Can you work these out from the model? Positions are in its coordinate system, mm. Give positions to 0.01 mm unless a question says otherwise; leave off trailing zeros. Order: outer loops, then holes, each group sorted by start corner. A loop starts at its lowest first (then second) coordinate and runs counter-clockwise, first axis right, second up. Notation, with made-up numbers: M 13.25,-12 L 24.25,-12 A23 cw 24.25,-4 Z; hole C -28,-16 d5. An arc over 180 degrees is marked long. Use one line per item in the form item = value. Start each with the question number.
1. Will these pins go through, and if not, where does the flat tip stop? P1, Ø3, axis at x = 86.5, y = 63.5, coming from the -Z side; P2, Ø2.5, axis at x = 24, y = 24, coming from the -Z side.
2. I want a section at B-B, the plane z = 2.2. Count the separate pieces of the cut face and the enclosed holes in it, and give its area (3 significant figures).
3. I want a section at A-A, the plane x = 36. List the corners of the cut face in (y, z) for me, and give its area (3 significant figures).
4. I want a section at C-C, the plane y = 80.5. List the corners of the cut face in (x, z) for me.
5. I need wall thicknesses on L1, parallel to X at y = 63.55, z = 1.6; L2, parallel to Y at x = 72, z = 2.8; L3, parallel to Y at x = 85.55, z = 1.9. Which ranges of each line are inside material? Lowest first, please.
6. I want a section at D-D, the plane x = 68. List the corners of the cut face in (y, z) for me.
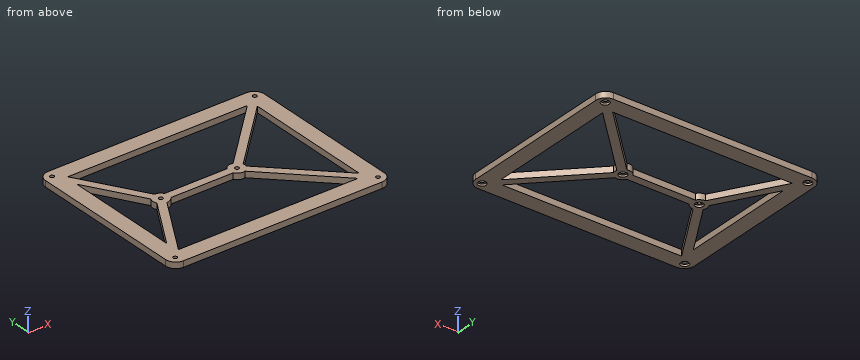
```python
from build123d import *

# Parameters (mm, degrees)
SKETCH002_R     = 1
PAD001_DEPTH    = 3
SKETCH003_R     = 2
POCKET001_DEPTH = 1


with BuildPart() as part:
    # Sketch002 → Pad001 (new body)
    with BuildSketch(Plane.XY):
        with BuildLine():
            Line((129.15, 25), (129.15, 102.15))
            ThreePointArc((129.15, 102.15), (127.685534, 105.685534), (124.15, 107.15))
            Line((124.15, 107.15), (25, 107.15))
            ThreePointArc((25, 107.15), (21.464466, 105.685534), (20, 102.15))
            Line((20, 102.15), (20, 25))
            ThreePointArc((20, 25), (21.464466, 21.464466), (25, 20))
            Line((25, 20), (124.15, 20))
            ThreePointArc((124.15, 20), (127.685534, 21.464466), (129.15, 25))
        make_face()
        with Locations((24, 103.15)):
            Circle(SKETCH002_R, mode=Mode.SUBTRACT)
        with Locations((24, 24)):
            Circle(SKETCH002_R, mode=Mode.SUBTRACT)
        with Locations((125.15, 24)):
            Circle(SKETCH002_R, mode=Mode.SUBTRACT)
        with Locations((125.15, 103.15)):
            Circle(SKETCH002_R, mode=Mode.SUBTRACT)
        with Locations((85.55, 63.55)):
            Circle(SKETCH002_R, mode=Mode.SUBTRACT)
        with Locations((47.5, 63.55)):
            Circle(SKETCH002_R, mode=Mode.SUBTRACT)
        with BuildLine():
            ThreePointArc((50.964102, 65.55), (49.479216, 67.026018), (47.452085, 67.549713))
            Line((28.699389, 99.15), (47.452085, 67.549713))
            Line((118.321573, 99.15), (28.699389, 99.15))
            Line((86.585276, 67.413703), (118.321573, 99.15))
            ThreePointArc((86.585276, 67.413703), (84.019266, 67.245518), (82.085898, 65.55))
            Line((50.964102, 65.55), (82.085898, 65.55))
        make_face(mode=Mode.SUBTRACT)
        with BuildLine():
            ThreePointArc((82.085898, 61.55), (84.020434, 59.853999), (86.587717, 59.686951))
            Line((118.314728, 28), (86.587717, 59.686951))
            Line((28.703156, 28), (118.314728, 28))
            Line((47.449866, 59.550314), (28.703156, 28))
            ThreePointArc((47.449866, 59.550314), (49.478252, 60.073433), (50.964102, 61.55))
            Line((50.964102, 61.55), (82.085898, 61.55))
        make_face(mode=Mode.SUBTRACT)
        with BuildLine():
            Line((89.414357, 62.517165), (121.15, 30.821592))
            Line((121.15, 30.821592), (121.15, 96.321573))
            Line((121.15, 96.321573), (89.413703, 64.585276))
            ThreePointArc((89.414357, 62.517165), (89.55, 63.551263), (89.413703, 64.585276))
        make_face(mode=Mode.SUBTRACT)
        with BuildLine():
            Line((44.012189, 65.508361), (28, 92.490603))
            Line((28, 92.490603), (28, 34.647227))
            Line((28, 34.647227), (44.011104, 61.593574))
            ThreePointArc((44.012189, 65.508361), (43.5, 63.551109), (44.011104, 61.593574))
        make_face(mode=Mode.SUBTRACT)
    extrude(amount=PAD001_DEPTH)

    # Sketch003 → Pocket001 (cut)
    with BuildSketch(Plane.XY):
        with Locations((24, 103.15)):
            Circle(SKETCH003_R)
        with Locations((24, 24)):
            Circle(SKETCH003_R)
        with Locations((125.15, 24)):
            Circle(SKETCH003_R)
        with Locations((125.15, 103.15)):
            Circle(SKETCH003_R)
        with Locations((85.55, 63.55)):
            Circle(SKETCH003_R)
        with Locations((47.5, 63.55)):
            Circle(SKETCH003_R)
    extrude(amount=POCKET001_DEPTH, mode=Mode.SUBTRACT)


solid = part.part
```
Check result:
q1.P1 = 0
q1.P2 = 1
q2.separate_pieces = 1
q2.enclosed_holes = 10
q2.area = 3,700 mm2
q3.outline = M 20,0 L 28,0 L 28,3 L 20,3 Z; M 40.28,0 L 48.11,0 L 48.11,3 L 40.28,3 Z; M 79.01,0 L 86.85,0 L 86.85,3 L 79.01,3 Z; M 99.15,0 L 107.15,0 L 107.15,3 L 99.15,3 Z
q3.area = 95.0 mm2
q4.outline = M 20,0 L 28,0 L 28,3 L 20,3 Z; M 35.12,0 L 39.77,0 L 39.77,3 L 35.12,3 Z; M 99.67,0 L 105.33,0 L 105.33,3 L 99.67,3 Z; M 121.15,0 L 129.15,0 L 129.15,3 L 121.15,3 Z
q5.L1 = 20 to 28, 43.5 to 46.5, 48.5 to 84.55, 86.55 to 89.55, 121.15 to 129.15
q5.L2 = 20 to 28, 61.55 to 65.55, 99.15 to 107.15
q5.L3 = 20 to 28, 59.55 to 62.55, 64.55 to 67.55, 99.15 to 107.15
q6.outline = M 20,0 L 28,0 L 28,3 L 20,3 Z; M 61.55,0 L 65.55,0 L 65.55,3 L 61.55,3 Z; M 99.15,0 L 107.15,0 L 107.15,3 L 99.15,3 Z
